Model file for the job. Use its own axes, mm. A direction names the side the tool comes from. Give positions to 0.01 mm unless a question says otherwise; leave off trailing zeros. Order: outer loops, then holes, each group sorted by start corner. A loop starts at its lowest first (then second) coordinate and runs counter-clockwise, first axis right, second up. Notation, with made-up numbers: (-22, 73) - (26, 73) arc R15 ccw to (26, 79) - close; hole circle Ø5 at (40.25, -18.75). An arc over 180 degrees is marked (long way). Return JSON: item names as keys, results as strings. Group by question number.
from build123d import *

# Parameters (mm, degrees)
F0_W          = 38.1
F0_H          = 609.6
F1_DEPTH      = 69.85
F1_DEPTH_BACK = 69.85
F2_W          = 88.9
F2_H          = 19.05
F3_DEPTH      = 38.1
F5_R          = 15.875
F6_DEPTH      = 50.8
F7_W          = 88.9
F7_H          = 19.05
F7_W_2        = 139.7
F7_H_2        = 76.2
F8_DEPTH      = 38.1
F9_R          = 6.35
F11_DEPTH     = 3.175
F12_R         = 6.35


with BuildPart() as f1:
    # F0 (on Front) → F1 (new body, two sides)
    with BuildSketch(Plane.XZ) as f1_sk:
        Rectangle(F0_W, F0_H)
    extrude(amount=F1_DEPTH)
    extrude(f1_sk.sketch, amount=-F1_DEPTH_BACK)

    # F2 (on face) → F3 (cut)
    with BuildSketch(Plane(origin=(-19.05, 0, 0), x_dir=(0, -1, 0), z_dir=(-1, 0, 0))):
        with Locations((-25.4, 269.875)):
            Rectangle(F2_W, F2_H)
    extrude(amount=-F3_DEPTH, mode=Mode.SUBTRACT)

    # F5 (on face) → F6 (cut)
    with BuildSketch(Plane(origin=(-19.05, 0, 0), x_dir=(0, -1, 0), z_dir=(-1, 0, 0))):
        with Locations((31.75, 209.55)):
            Circle(F5_R)
        with Locations((-31.75, 107.95)):
            Circle(F5_R)
        with Locations((31.75, -50.8)):
            Circle(F5_R)
        with Locations((-31.75, -152.4)):
            Circle(F5_R)
    extrude(amount=-F6_DEPTH, mode=Mode.SUBTRACT)

    # F7 (on face) → F8 (cut, through all)
    with BuildSketch(Plane.YZ.offset(19.05)):
        with Locations((25.4, 9.525)):
            Rectangle(F7_W, F7_H)
        with Locations((0, -266.7)):
            Rectangle(F7_W_2, F7_H_2)
    extrude(amount=-F8_DEPTH, mode=Mode.SUBTRACT)

    # F9
    f9_edges = [f1.edges().sort_by_distance(p)[0] for p in [
        (-19.05, -15.875, 209.55),
        (-19.05, 47.625, 107.95),
        (19.05, -15.875, -50.8),
        (19.05, 47.625, -152.4),
    ]]
    fillet(f9_edges, radius=F9_R)

    # F10 (on face) → F11 (cut)
    with BuildSketch(Plane(origin=(0, 69.85, 0), x_dir=(-1, 0, 0), z_dir=(0, 1, 0))):
        with BuildLine():
            ThreePointArc((6.5330743462, 224.4064063608), (-1.0936353663, 230.8472931087), (-6.1669256538, 222.25))
            Line((-6.1669256538, 222.25), (-6.1669256538, 190.5))
            ThreePointArc((-6.1669256538, 190.5), (0.1830743462, 184.15), (6.5330743462, 190.5))
            Line((6.5330743462, 190.5), (6.5330743462, 224.4064063608))
        make_face()
        with BuildLine():
            ThreePointArc((6.7926369745, -50.8), (1.5520159153, -44.3027542125), (-5.9073630255, -48.0492162406))
            Line((-5.9073630255, -48.0492162406), (-5.9073630255, -79.7992162406))
            ThreePointArc((-5.9073630255, -79.7992162406), (1.733975859, -83.0137515295), (6.7926369745, -76.4461610438))
            Line((6.7926369745, -76.4461610438), (6.7926369745, -50.8))
        make_face()
    extrude(amount=-F11_DEPTH, mode=Mode.SUBTRACT)

    # F12
    f12_edges = [f1.edges().sort_by_distance(p)[0] for p in [
        (19.05, -69.85, 38.1),
        (-19.05, -69.85, 38.1),
        (0, -69.85, 304.8),
        (0, -69.85, -228.6),
    ]]
    fillet(f12_edges, radius=F12_R)


solid = f1.part
(1) Drop flat-ended pins along their axis: pin 1 Ø19 at (y, z) = (-31.75, 209.55) entering from +X; pin 2 Ø4 at (x, z) = (-1, -65.5) entering from +Y (3 decimals); pin 3 Ø15 at (x, z) = (4, 271) entering from +Y. Give the stop position or say it passes through.
(2) Slice it at A-A (y = -31.75). Give the cut face in (x, z) (3 decimals), and give its area (3 significant figures).
(3) Slice it at C-C (y = 31.75). Give the cut face in (x, z) (3 decimals).
(4) 3-axis set-ups, long thin cutter, end or side, ignore diameter. For faces 4 (the face through (0.94, 68.28, 230.87)), 5 (the face through (2.95, -29.68, 225.29)), 6 (the face through (0, 25, 0)): which of +Z, -Z, +X, -X, +Y, -Y reach the whole face in a straight line?
(5) Slice it at B-B (z = -152.4). Give the cut face in (x, y) (3 decimals).
(6) Pull direction Y, two halves, no side cores. Call faces 1 (the face through (0, 2, 304.8)), 2 (the face through (-3.4, -20.05, -40.07)), 3 (the face through (0, 66.675, -63)): released by +Y, released by -Y, zero draft, split by the parting line, or undercut.
(7) Drill centre lines: L1, parallel to Z at x = 1, y = 4.5; L2, parallel to Z at x = 5, y = -31; L3, parallel to Z at x = 9, y = 33.5. Where is each one in solid material? Low to high.
(8) Slice it at D-D (x = 0). Give the cut face in (y, z) (3 decimals), and give its area (3 significant figures).
Result set:
{
 "1": {"pin 1": "passes through", "pin 2": "stops at y = 66.675", "pin 3": "stops at y = -19.05"},
 "2": {"outline": "(-19.05, -228.6) - (19.05, -228.6) - (19.05, -73.025) arc R6.35 ccw to (12.7, -66.675) - (-19.05, -66.675) - close; (-19.05, -34.925) - (12.7, -34.925) arc R6.35 ccw to (19.05, -28.575) - (19.05, 193.675) - (-12.7, 193.675) arc R6.35 ccw to (-19.05, 187.325) - close; (-19.05, 231.775) arc R6.35 ccw to (-12.7, 225.425) - (19.05, 225.425) - (19.05, 304.8) - (-19.05, 304.8) - close", "area": "17,900 mm²"},
 "3": {"outline": "(-19.05, -228.6) - (19.05, -228.6) - (19.05, -174.625) arc R6.35 ccw to (12.7, -168.275) - (-19.05, -168.275) - close; (-19.05, -136.525) - (12.7, -136.525) arc R6.35 ccw to (19.05, -130.175) - (19.05, 0) - (-19.05, 0) - close; (-19.05, 19.05) - (19.05, 19.05) - (19.05, 92.075) - (-12.7, 92.075) arc R6.35 ccw to (-19.05, 85.725) - close; (-19.05, 130.175) arc R6.35 ccw to (-12.7, 123.825) - (19.05, 123.825) - (19.05, 260.35) - (-19.05, 260.35) - close; (-19.05, 279.4) - (19.05, 279.4) - (19.05, 304.8) - (-19.05, 304.8) - close"},
 "4": {"face 4": "+Y", "face 5": "+X, -X", "face 6": "+X, -X, +Y"},
 "5": {"outline": "(-19.05, -63.5) arc R6.35 ccw to (-12.7, -69.85) - (12.7, -69.85) arc R6.35 ccw to (19.05, -63.5) - (19.05, 9.525) arc R6.35 ccw to (12.7, 15.875) - (-19.05, 15.875) - close; (-19.05, 47.625) - (12.7, 47.625) arc R6.35 ccw to (19.05, 53.975) - (19.05, 69.85) - (-19.05, 69.85) - close"},
 "6": {"face 1": "zero draft", "face 2": "undercut", "face 3": "released by +Y"},
 "7": {"L1": "z = -228.6 to 0, 19.05 to 260.35, 279.4 to 304.8", "L2": "z = -228.6 to -66.66, -34.94 to 193.69, 225.41 to 304.8", "L3": "z = -228.6 to -168.18, -136.62 to 0, 19.05 to 92.17, 123.73 to 260.35, 279.4 to 304.8"},
 "8": {"outline": "(-69.85, -222.25) arc R6.35 ccw to (-63.5, -228.6) - (69.85, -228.6) - (69.85, -83.239) - (66.675, -83.239) - (66.675, -44.154) - (69.85, -44.154) - (69.85, 0) - (-19.05, 0) - (-19.05, 19.05) - (69.85, 19.05) - (69.85, 184.153) - (66.675, 184.153) - (66.675, 230.939) - (69.85, 230.939) - (69.85, 260.35) - (-19.05, 260.35) - (-19.05, 279.4) - (69.85, 279.4) - (69.85, 304.8) - (-63.5, 304.8) arc R6.35 ccw to (-69.85, 298.45) - close; hole circle Ø31.75 at (-31.75, -50.8); hole circle Ø31.75 at (-31.75, 209.55); hole circle Ø31.75 at (31.75, -152.4); hole circle Ø31.75 at (31.75, 107.95)", "area": "67,700 mm²"}
}
